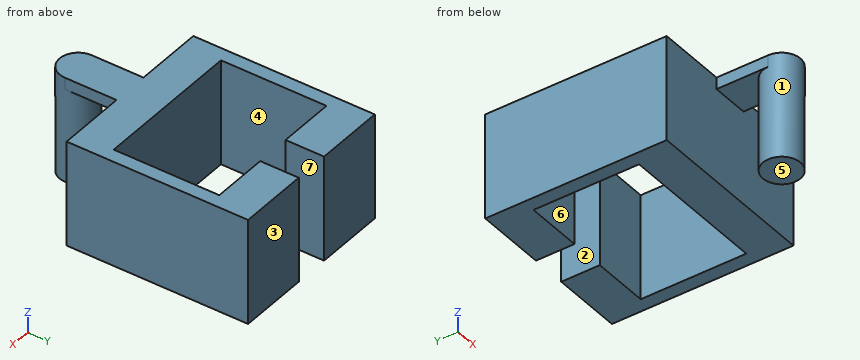
```python
from build123d import *

# Parameters (mm, degrees)
SKETCH1_R            = 6.7564
BOSS_EXTRUDE2_DEPTH  = 38.1
SKETCH2_W            = 13.5128
SKETCH2_H            = 18.6436
BOSS_EXTRUDE3_DEPTH  = 4.23926
BOSS_EXTRUDE6_DEPTH  = 13.49502
SKETCH7_W            = 4.8768
SKETCH7_H            = 38.1
BOSS_EXTRUDE10_DEPTH = 38.1
SKETCH8_W            = 25.4
SKETCH8_H            = 38.1
BOSS_EXTRUDE11_DEPTH = 13.91158


with BuildPart() as part:
    # Sketch1 → Boss-Extrude2 (new body)
    with BuildSketch(Plane.XY):
        with Locations(Location((0, 0, 0), (0, 0, 180))):
            Circle(SKETCH1_R)
    extrude(amount=BOSS_EXTRUDE2_DEPTH)

    # Sketch2 → Boss-Extrude3 (add)
    with BuildSketch(Plane.XY.offset(38.1)):
        with Locations((0, 9.3218)):
            Rectangle(SKETCH2_W, SKETCH2_H)
    extrude(amount=-BOSS_EXTRUDE3_DEPTH)

    # Sketch4 → Boss-Extrude6 (add)
    with BuildSketch(Plane(origin=(0, 18.6436, 0), x_dir=(1, 0, 0), z_dir=(0, 1, 0))):
        Polygon((0, -38.1), (-31.75, -38.1), (-31.75, 0), (31.75, 0), (31.75, -38.1), align=None)
    extrude(amount=BOSS_EXTRUDE6_DEPTH)

    # Sketch7 → Boss-Extrude10 (add)
    with BuildSketch(Plane(origin=(0, 32.13862, 0), x_dir=(1, 0, 0), z_dir=(0, 1, 0))):
        with Locations((-29.3116, -19.05)):
            Rectangle(SKETCH7_W, SKETCH7_H)
        with Locations((29.3116, -19.05)):
            Rectangle(SKETCH7_W, SKETCH7_H)
    extrude(amount=BOSS_EXTRUDE10_DEPTH)

    # Sketch8 → Boss-Extrude11 (add)
    with BuildSketch(Plane(origin=(0, 70.23862, 0), x_dir=(1, 0, 0), z_dir=(0, 1, 0))):
        with Locations((-19.05, -19.05)):
            Rectangle(SKETCH8_W, SKETCH8_H)
        with Locations((19.05, -19.05)):
            Rectangle(SKETCH8_W, SKETCH8_H)
    extrude(amount=BOSS_EXTRUDE11_DEPTH)


solid = part.part
```
CAD build for the part. Positions are in the model's coordinates, mm. Face numbers are marked on the shaded views. A direction names the side the tool comes from. Give positions to 0.01 mm unless a question says otherwise; leave off trailing zeros. Write each loop counter-clockwise with the first axis right and the second up, starting at its lowest first coordinate (ties: lowest second). Pieces come first, ordered by that corner, then holes. Notation, with made-up numbers: M -19,-11 L 16,-11 A13 cw 16,1 Z; hole C 88,58 d6. An arc over 180 degrees is marked long. Return JSON: item names as keys, results as strings. Group by question number.
(1) Band-saw the part on B-B (x = 17.5). Give the cut face in (y, z).
(2) Band-saw the part on D-D (x = 0). Give the cut face in (y, z), and give its area (3 significant figures).
(3) Flat gauge pins, fed straight in: pin 1 Ø8 at (x, z) = (2, 18.5) entering from +Y; pin 2 Ø1.3 at (y, z) = (5, 36.5) entering from +X; pin 3 Ø7 at (x, y) = (-1.5, 12) entering from -Z. Where does each tip first touch, or does it go through?
(4) 3-axis set-ups, long thin cutter, end or side, ignore diameter. For the marked faces 5, 6 and 7: which of +Z, -Z, +X, -X, +Y, -Y reach the whole face in a straight line?
(5) Band-saw the part on C-C (z = 24.5). Give the cut face in (x, y).
(6) Drill centre lines: L1, parallel to X at y = 74.5, z = 32.5; L2, parallel to Y at x = 24.5, z = 34.5; L3, parallel to X at y = 52.5, z = 22. Where is each one in solid material? Low to high. Write a range as [from, to].
(7) Mould opens along X. For the marked faces 1, 2, 3 and 4 say: pulls with the +X half, pulls with the -X half, needs draft (parallel to the pull), parting line crosses it, or undercut.
(8) Band-saw the part on A-A (y = 43). Give the cut face in (x, z), and give its area (3 significant figures).
Entries:
{
 "1": {"outline": "M 18.64,0 L 32.14,0 L 32.14,38.1 L 18.64,38.1 Z; M 70.24,0 L 84.15,0 L 84.15,38.1 L 70.24,38.1 Z"},
 "2": {"outline": "M -6.76,0 L 6.76,0 L 6.76,33.86 L 18.64,33.86 L 18.64,0 L 32.14,0 L 32.14,38.1 L -6.76,38.1 Z", "area": "1,080 mm^2"},
 "3": {"pin 1": "stops at y = 32.14", "pin 2": "stops at x = 6.76", "pin 3": "stops at z = 33.86"},
 "4": {"face 5": "-Z, +X, -X, +Y, -Y", "face 6": "+Z, -Z", "face 7": "+Z, -Z, +Y"},
 "5": {"outline": "M -31.75,18.64 L 31.75,18.64 L 31.75,84.15 L 6.35,84.15 L 6.35,70.24 L 26.87,70.24 L 26.87,32.14 L -26.87,32.14 L -26.87,70.24 L -6.35,70.24 L -6.35,84.15 L -31.75,84.15 Z; C 0,0 d13.51"},
 "6": {"L1": "x = [-31.75, -6.35], [6.35, 31.75]", "L2": "y = [18.64, 32.14], [70.24, 84.15]", "L3": "x = [-31.75, -26.87], [26.87, 31.75]"},
 "7": {"face 1": "parting line crosses it", "face 2": "undercut", "face 3": "needs draft", "face 4": "undercut"},
 "8": {"outline": "M -31.75,0 L -26.87,0 L -26.87,38.1 L -31.75,38.1 Z; M 26.87,0 L 31.75,0 L 31.75,38.1 L 26.87,38.1 Z", "area": "372 mm^2"}
}
